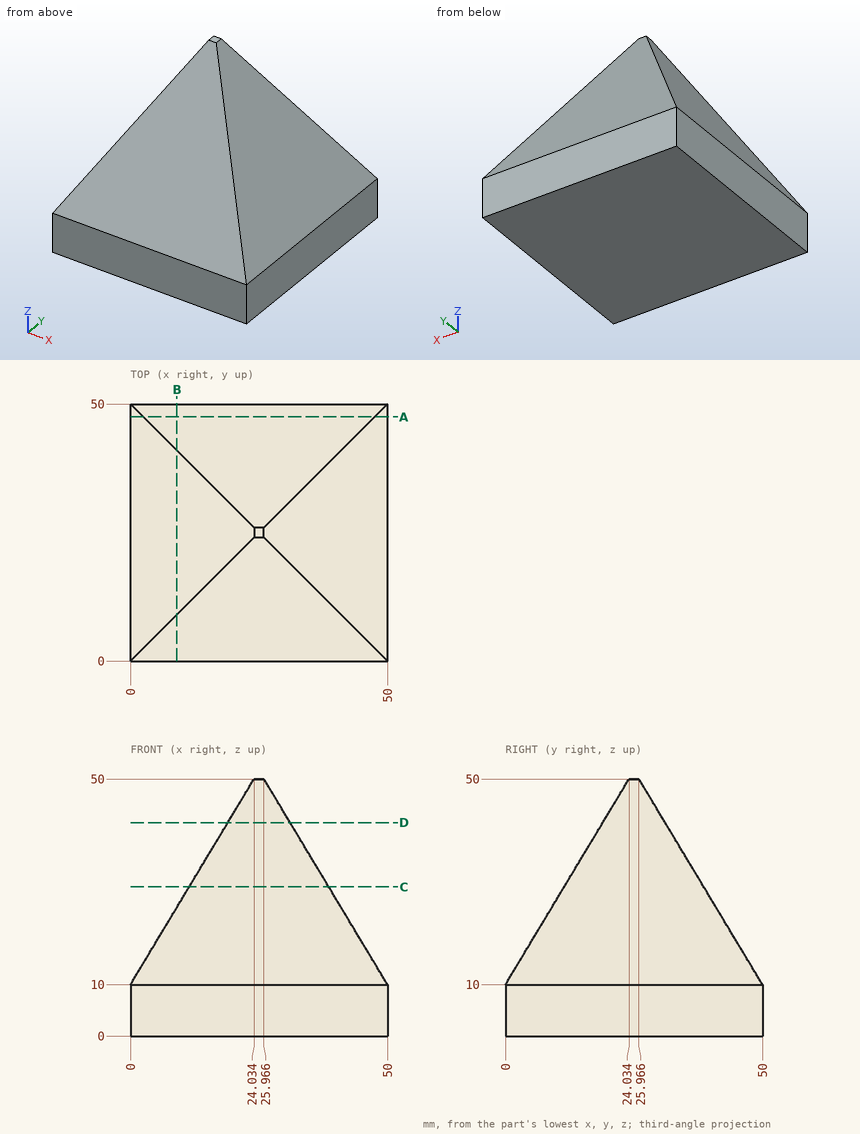
Drawing for the job (mm, zero at the part's lowest x, y, z). Round coordinates to 2 decimals unless told otherwise and drop trailing zeros. Loops run counter-clockwise (first coordinate to the right, second up) from the corner with the lowest first, then second, coordinate; pieces in that order, holes last. Notation, with made-up numbers: M 1,-8.75 L 26,-8.75 A22 cw 26,2.25 Z; hole C -17,-27 d6. An arc over 180 degrees is marked long. Use a Markdown table: item, result. Add a question column.
(1) Cut at C-C (z = 29). Give the cut face in (x, y), and give its area (3 significant figures).
(2) Cut at A-A (y = 47.5). Give the cut face in (x, z).
(3) Cut at D-D (z = 41.5). Give the cut face in (x, y).
(4) Cut at B-B (x = 9). Give the cut face in (y, z), and give its area (3 significant figures).
(5) Flat gauge pins, fed straight in: pin 1 (10 mm diameter, centred on y = 23.5, z = 43, fed in from -X) (1 decimal); pin 2 (10 mm diameter, centred on y = 5.5, z = 18.5, fed in from -X); pin 3 (5 mm diameter, centred on x = 32, z = 13.5, fed in from -Y). Where does each tip first touch, or does it go through?
(6) Drill centre lines: line 1 (X direction, y = 33, z = 19); line 2 (X direction, y = 35.5, z = 11); line 3 (Z direction, x = 10.5, y = 32) (1 decimal). Where is each one in solid material? Low to high.
Geometry says:
| question | item | result |
|---|---|---|
| 1 | outline | M 11.42,11.42 L 38.58,11.42 L 38.58,38.58 L 11.42,38.58 Z |
| 1 | area | 738 mm² |
| 2 | outline | M 0,0 L 50,0 L 50,10 L 47.5,14.16 L 2.5,14.16 L 0,10 Z |
| 3 | outline | M 18.93,18.93 L 31.07,18.93 L 31.07,31.07 L 18.93,31.07 Z |
| 4 | outline | M 0,0 L 50,0 L 50,10 L 41,24.98 L 9,24.98 L 0,10 Z |
| 4 | area | 1,110 mm² |
| 5 | pin 1 | stops at x = 16.8 |
| 5 | pin 2 | stops at x = 2.1 |
| 5 | pin 3 | stops at y = 0.6 |
| 6 | line 1 | x = 5.41 to 44.59 |
| 6 | line 2 | x = 0.6 to 49.4 |
| 6 | line 3 | z = 0 to 27.5 |
